Input: part model. Units: mm. Frame: model coordinates. A direction names the side the tool comes from. Coordinates: 2 decimals unless noted, no trailing zeros. Order: outer loops, then holes, each group sorted by start corner. A loop starts at its lowest first (then second) coordinate and runs counter-clockwise, first axis right, second up. Notation, with made-up numbers: M -25,28 L -1,28 A22 ccw -1,38 Z; hole C -11.75,12 d2. An arc over 180 degrees is marked long. One line per item, written item: value.
```python
from build123d import *

# Parameters (mm, degrees)
F1_DEPTH = 1.27
F2_DEPTH = 4.445
F3_SIZE2 = 0.762
F3_SIZE  = 0.762


# Not quite as in the source:
# - a feature names something its author has since deleted; it is built from what else it names


with BuildPart() as f1:
    # F0 (on Front) → F1 (new body)
    with BuildSketch(Plane.XZ):
        with BuildLine():
            Line((-8.6160342025, -3.05308), (-25.146, -3.05308))
            ThreePointArc((-25.146, -3.05308), (-25.0213724382, -4.0720308287), (-24.855468258, -5.08508))
            Line((-24.855468258, -5.08508), (-19.05, -5.08508))
            Line((-19.05, -5.08508), (-19.05, -7.37108))
            Line((-19.05, -7.37108), (-24.3224034139, -7.37108))
            ThreePointArc((-24.3224034139, -7.37108), (-0.002803144, -25.7679203368), (24.3167971258, -7.37108))
            Line((24.3167971258, -7.37108), (19.05, -7.37108))
            Line((19.05, -7.37108), (19.05, -5.08508))
            Line((19.05, -5.08508), (24.8498619699, -5.08508))
            ThreePointArc((24.8498619699, -5.08508), (25.0157661502, -4.0720308287), (25.1403937119, -3.05308))
            Line((25.1403937119, -3.05308), (8.6160342025, -3.05308))
            ThreePointArc((8.6160342025, -3.05308), (11.5583898274, -7.2348059893), (12.5961765249, -12.2415302321))
            ThreePointArc((12.5961765249, -12.2415302321), (-5.0067242428, -23.7999200595), (-8.6160342025, -3.05308))
        make_face()
        with BuildLine():
            Line((8.6160342025, -3.05308), (-8.6160342025, -3.05308))
            ThreePointArc((-8.6160342025, -3.05308), (-5.0067242428, -23.7999200595), (12.5961765249, -12.2415302321))
            ThreePointArc((12.5961765249, -12.2415302321), (11.5583898274, -7.2348059893), (8.6160342025, -3.05308))
        make_face()
        with BuildLine():
            ThreePointArc((8.6160342025, -3.05308), (0, 0.3546462928), (-8.6160342025, -3.05308))
            Line((-8.6160342025, -3.05308), (8.6160342025, -3.05308))
        make_face()
    extrude(amount=F1_DEPTH)

    # F0 (on Front) → F2 (join)
    with BuildSketch(Plane.XZ):
        with BuildLine():
            Line((-19.05, -5.08508), (-24.855468258, -5.08508))
            ThreePointArc((-24.855468258, -5.08508), (-24.6154903144, -6.2342721517), (-24.3224034139, -7.37108))
            Line((-24.3224034139, -7.37108), (-19.05, -7.37108))
            Line((-19.05, -7.37108), (-19.05, -5.08508))
        make_face()
        with BuildLine():
            Line((19.05, -7.37108), (24.3167971258, -7.37108))
            ThreePointArc((24.3167971258, -7.37108), (24.6098840263, -6.2342721517), (24.8498619699, -5.08508))
            Line((24.8498619699, -5.08508), (19.05, -5.08508))
            Line((19.05, -5.08508), (19.05, -7.37108))
        make_face()
    extrude(amount=F2_DEPTH)

    # F3
    f3_edges = [f1.edges().sort_by_distance(p)[0] for p in [
        (21.949931, -4.445, -5.08508),
        (19.05, -4.445, -6.22808),
        (21.683399, -4.445, -7.37108),
        (24.609884, -4.445, -6.234272),
        (-21.686202, -4.445, -7.37108),
        (-24.61549, -4.445, -6.234272),
        (-19.05, -4.445, -6.22808),
        (-21.952734, -4.445, -5.08508),
    ]]
    chamfer(f3_edges, length=F3_SIZE, length2=F3_SIZE2)


solid = f1.part
```
(1) Ray query, line 1 (Y direction, x = -14, z = -9.25); line 2 (X direction, y = -1.95, z = -5.75); line 3 (Z direction, x = 21.5, y = -3.35). Return the intervals inside material, ascending. Write a range as from..to.
Data:
line 1: y = -1.27..0
line 2: x = -24.72..-19.05, 19.05..24.72
line 3: z = -7.37..-5.09
(2) Cut plane B-B on x = -22. Output: boundary loops of the cut face in (y, z) (3 decimals).
Data:
outline: M -4.445,-6.609 L -3.683,-7.371 L -1.27,-7.371 L -1.27,-12.939 L 0,-12.939 L 0,-3.053 L -1.27,-3.053 L -1.27,-5.085 L -3.683,-5.085 L -4.445,-5.847 Z
(3) Cut plane D-D on x = -5. Output: boundary loops of the cut face in (y, z), plus the area to 3 significant figures.
Data:
outline: M -1.27,-25.27 L 0,-25.27 L 0,-0.68 L -1.27,-0.68 Z
area: 31.2 mm2
(4) Draft query along X for faces 4 (the flat face through (19.05, -2, -6)), 5 (the cylindrical face through (0.133, -0.626, 0.354)), 6 (the flat face through (17, -1, -3.053)). Return one class per face: released by +X, released by -X, zero draft, split by the parting line, or undercut.
Data:
face 4: undercut
face 5: split by the parting line
face 6: zero draft
(5) Access query for faces 1 (the flat face through (-22, -2, -7.371)), 2 (the flat face through (-17, -1, -3.053)), 3 (the flat face through (22, -2, -5.085)). Directions: +Z, -Z, +X, -X, +Y, -Y. A direction counts if a zero-diameter tool reaches every point of the face in a straight line with its end or side. Return the directions, or none.
Data:
face 1: -Z, +X, -X, -Y
face 2: +Z, -X, +Y, -Y
face 3: +Z, +X, -X, -Y
(6) Cut plane C-C on z = -21. Output: boundary loops of the cut face in (x, y).
Data:
outline: M -14.78,-1.27 L 14.77,-1.27 L 14.77,0 L -14.78,0 Z
(7) Cut plane A-A on y = -1.9. Output: boundary loops of the cut face in (x, z).
Data:
outline: M -24.86,-5.09 A25.27 ccw -24.32,-7.37 L -19.05,-7.37 L -19.05,-5.09 Z; M 19.05,-7.37 L 24.32,-7.37 A25.27 ccw 24.85,-5.09 L 19.05,-5.09 Z
(8) First-contact query: pin 1 (1 mm diameter, centred on x = -6, z = -19, fed in from -Y); pin 2 (1.4 mm diameter, centred on x = 17, y = -1, fed in from +Z); pin 3 (1.1 mm diameter, centred on y = -3, z = -5.5, fed in from +X). Flat tips, straight axial feed; report the tip coordinate or a pass-through.
Data:
pin 1: stops at y = -1.27
pin 2: stops at z = -3.05
pin 3: stops at x = 24.85
